Autodesk Inventor part; units mm, degrees
ref_plane "YZ Plane" through (0, 0, 0) normal (1, 0, 0) x (0, 1, 0)
ref_plane "XZ Plane" through (0, 0, 0) normal (0, 1, 0) x (-1, 0, 0)
ref_plane "XY Plane" through (0, 0, 0) normal (0, 0, 1) x (1, 0, 0)
sketch "Esboço1" plane through (0, 0, 0) normal (0, 0, 1) x (1, 0, 0)
  line L0 (-20, -59.85) -> (20, -59.85)
  line L1 (20, -59.85) -> (20, 59.85)
  line L2 (20, 59.85) -> (-20, 59.85)
  line L3 (-20, 59.85) -> (-20, -59.85)
  line L4 (-20, 59.85) -> (20, 59.85)
  circle A0 centre (0, 49.85) radius 5 construction
  circle A1 centre (0, 49.85) radius 28 construction
  circle A2 centre (0, 49.85) radius 74 construction
  line L5 (-20, 30.2541) -> (20, 30.2541) construction
  line L6 (-20, -24.15) -> (20, -24.15) construction
  line L7 (-103.6, 0) -> (103.6, 0) construction
  line L8 (0, -96.59) -> (0, 160.59) construction
  line L9 (-20, 36.756) -> (20, 59.85)
  point P0 (0, 0)
  dimension "d0" = 119.7
  dimension "d1" = 40
  dimension "d41" = 10
  dimension "d42" = 109.7
  dimension "d43" = 56
  dimension "d45" = 84
  dimension "d49" = 30
  dimension "d58" = 10
extrude "Extrusão1" add sketch "Esboço1" along normal mid plane 10
extrude "Extrusão4" cut sketch "Esboço1" along normal through all both and the other way through all contours L3 L2 L9
sketch "Esboço2" plane through (-20, -59.85, -5) normal (0, -1, 0) x (1, 0, 0)
  line L0 (40, 10) -> (40, 0)
  line L1 (40, 5) -> (0, 5) construction
  line L2 (0, 0) -> (0, 10)
  line L3 (0, 0) -> (0, 10)
  line L4 (40, 0) -> (40, 10)
  line L5 (0, 10) -> (40, 10) construction
  line L6 (20, 10) -> (20, 0) construction
  line L7 (40, 0) -> (0, 0) construction
  point P0 (20, 5)
  point P1 (7.5, 5)
  point P2 (32.5, 5)
  dimension "d9" = 7.5
  dimension "d10" = 7.5
  dimension "d37" = 25
hole "Furo1" at (-12.5, -59.85, 0) at (12.5, -59.85, 0) direction (0, 1, 0) diameter 3.242 depth 15 tip angle 118
sketch "Esboço3" plane through (0, 0, 5) normal (0, 0, 1) x (1, 0, 0)
  point P0 (0, 0)
  point P1 (0, 37.5)
  point P2 (0, 49.85)
hole "Furo2" [suppressed]
sketch "Esboço6" plane through (20, 59.85, 5) normal (-0.5, 0.8660254, 0) x (0.8660254, 0.5, 0)
  line L0 (0, 0) -> (0, 10) construction
  line L1 (0, 5) -> (-46.188, 5) construction
  line L2 (-46.188, 0) -> (-46.188, 10) construction
  line L3 (-23.094, 5) -> (-23.094, 0) construction
  point P0 (-47.2455, 5)
  point P1 (-33.094, 5)
  point P2 (-13.094, 5)
  dimension "d50" = 20
hole "Furo3" at (-8.6603, 43.303, 0) direction (0.5, -0.8660254, 0) diameter 3.242 depth 15 tip angle 118 countersink diameter 10 countersink angle 90
properties part number "GRJ-03-116A" material "Fenolite OR"
Geometry: final body of the model. Coordinates: model frame, mm. A direction names the side the tool comes from. Round coordinates to 2 decimals unless told otherwise and drop trailing zeros. Order: outer loops, then holes, each group sorted by start corner. A loop starts at its lowest first (then second) coordinate and runs counter-clockwise, first axis right, second up. Notation, with made-up numbers: (14, -6.75) -> (23, -6.75) arc R21 cw to (23, 7.25) -> close; hole circle Ø3 at (73, 52.25). An arc over 180 degrees is marked (long way). Use one line per item in the form item = value.
(1) Section B-B on x = 15.5. Return loops of the section in (y, z), and give its area (3 significant figures).
Results list:
outline = (-59.85, -5) -> (57.25, -5) -> (57.25, 5) -> (-59.85, 5) -> close
area = 1,170 mm^2
(2) Ray query, probe 1 along X at (y, z) = (-48.25, 0); probe 2 along Z at (x, y) = (-12.5, -56.5); probe 3 along Z at (x, y) = (12, -52). Return the intervals inside material, ascending. Write a range as [from, to].
Results list:
probe_1 = [-20, -14.12], [-10.88, 10.88], [14.12, 20]
probe_2 = [-5, -1.62], [1.62, 5]
probe_3 = [-5, -1.54], [1.54, 5]
(3) Access query for faces 1 (the face through (20, -1, 0)), 2 (the face through (10.893, -52.245, 0.211)), 3 (the face through (-0.68, 29.66, 0.27)). Directions: +Z, -Z, +X, -X, +Y, -Y. A direction counts if a zero-diameter tool reaches every point of the face in a straight line with its end or side. Return the directions, or none.
Results list:
face_1 = +Z, -Z, +X, +Y, -Y
face_2 = -Y
face_3 = none
(4) Section A-A on x = 2.5. Return loops of the section in (y, z), and give its area (3 significant figures).
Results list:
outline = (-59.85, -5) -> (49.75, -5) -> (49.75, 5) -> (-59.85, 5) -> close
area = 1,100 mm^2
(5) First-contact query: pin 1 Ø1.9 at (x, z) = (12.5, 0) entering from +Y; pin 2 Ø2 at (x, z) = (-4.5, -3) entering from +Y; pin 3 Ø2.5 at (x, z) = (-12.5, 0) entering from -Y. Flat tips, straight axial feed; report the tip coordinate or a pass-through.
Results list:
pin_1 = 56.07
pin_2 = 46.28
pin_3 = -44.63
(6) Draft query along X for faces 4 (the face through (0, 1, -5)), 5 (the face through (-7.684, 40.209, 1.693)), 6 (the face through (-20, -11, 0)). Return one class per face: pulls with the +X half, pulls with the -X half, needs draft (parallel to the pull), parting line crosses it, or undercut.
Results list:
face_4 = needs draft
face_5 = undercut
face_6 = pulls with the -X half
